Could you check a few things on this model? Use its own coordinates, in mm. Coordinates: 2 decimals unless noted, no trailing zeros. Loops run counter-clockwise (first coordinate to the right, second up) from the corner with the lowest first, then second, coordinate; pieces in that order, holes last. Notation, with made-up numbers: (6, 44) -> (26, 44) arc R24 cw to (26, 80) -> close; hole circle Ø10 at (40, -32). An arc over 180 degrees is marked (long way). One line per question, with ' | ' between items.
from build123d import *

# Parameters (mm, degrees)
BOSS_EXTRUDE1_DEPTH = 6
SKETCH2_R           = 3.25
CUT_EXTRUDE1_DEPTH  = 82.391031447
SKETCH3_R           = 5.5
CUT_EXTRUDE2_DEPTH  = 4.8


with BuildPart() as part:
    # Sketch1 → Boss-Extrude1 (new body)
    with BuildSketch(Plane(origin=(0, 0, 0), x_dir=(1, 0, 0), z_dir=(0, 1, 0))):
        with BuildLine():
            Line((-36.5, -72.5), (36.5, -72.5))
            Line((36.5, -72.5), (36.5, -24.5))
            Line((36.5, -24.5), (26.5, -24.5))
            ThreePointArc((26.5, -24.5), (22.964466094, -23.035533906), (21.5, -19.5))
            Line((21.5, -19.5), (21.5, 37.5))
            ThreePointArc((21.5, 37.5), (22.964466094, 41.035533906), (26.5, 42.5))
            Line((26.5, 42.5), (36.5, 42.5))
            Line((36.5, 42.5), (36.5, 72.5))
            Line((36.5, 72.5), (-36.5, 72.5))
            Line((-36.5, 72.5), (-36.5, 42.5))
            Line((-36.5, 42.5), (-26.5, 42.5))
            ThreePointArc((-26.5, 42.5), (-22.964466094, 41.035533906), (-21.5, 37.5))
            Line((-21.5, 37.5), (-21.5, -19.5))
            ThreePointArc((-21.5, -19.5), (-22.964466094, -23.035533906), (-26.5, -24.5))
            Line((-26.5, -24.5), (-36.5, -24.5))
            Line((-36.5, -24.5), (-36.5, -72.5))
        make_face()
    extrude(amount=BOSS_EXTRUDE1_DEPTH)

    # Sketch2 → Cut-Extrude1 (cut, through all)
    with BuildSketch(Plane(origin=(0, 6, 0), x_dir=(1, 0, 0), z_dir=(0, 1, 0))):
        with Locations(Location((-30, 66, 0), (0, 0, 270))):
            Circle(SKETCH2_R)
        with Locations(Location((-30, 50, 0), (0, 0, 270))):
            Circle(SKETCH2_R)
        with Locations(Location((30, 50, 0), (0, 0, 90))):
            Circle(SKETCH2_R)
        with Locations(Location((30, 66, 0), (0, 0, 90))):
            Circle(SKETCH2_R)
        with Locations(Location((30, -50, 0), (0, 0, 270))):
            Circle(SKETCH2_R)
        with Locations(Location((30, -66, 0), (0, 0, 270))):
            Circle(SKETCH2_R)
        with Locations(Location((-30, -50, 0), (0, 0, 90))):
            Circle(SKETCH2_R)
        with Locations(Location((-30, -66, 0), (0, 0, 90))):
            Circle(SKETCH2_R)
    extrude(amount=-CUT_EXTRUDE1_DEPTH, mode=Mode.SUBTRACT)

    # Sketch3 → Cut-Extrude2 (cut)
    with BuildSketch(Plane(origin=(0, 6, 0), x_dir=(1, 0, 0), z_dir=(0, 1, 0))):
        with Locations(Location((-30, 50, 0), (0, 0, 270))):
            Circle(SKETCH3_R)
        with Locations(Location((30, 50, 0), (0, 0, 90))):
            Circle(SKETCH3_R)
        with Locations(Location((30, -50, 0), (0, 0, 270))):
            Circle(SKETCH3_R)
        with Locations(Location((-30, -50, 0), (0, 0, 90))):
            Circle(SKETCH3_R)
    extrude(amount=-CUT_EXTRUDE2_DEPTH, mode=Mode.SUBTRACT)


solid = part.part
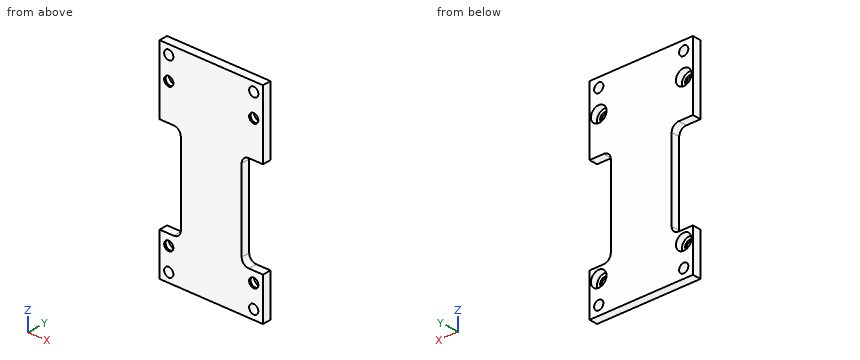
1) If we section it at D-D on z = 50: Please give me the cut outline in (x, y).
Data:
outline: (-36.5, 0) -> (-33.25, 0) -> (-33.25, 1.2) -> (-35.5, 1.2) -> (-35.5, 6) -> (-36.5, 6) -> close; (-26.75, 0) -> (26.75, 0) -> (26.75, 1.2) -> (24.5, 1.2) -> (24.5, 6) -> (-24.5, 6) -> (-24.5, 1.2) -> (-26.75, 1.2) -> close; (33.25, 0) -> (36.5, 0) -> (36.5, 6) -> (35.5, 6) -> (35.5, 1.2) -> (33.25, 1.2) -> close
2) If we section it at B-B on x = 30: Give the number of separate pieces and of enclosed holes in the cut face, and give its area (3 significant figures).
Data:
separate pieces: 6 | enclosed holes: 0 | area: 269 mm²
3) I need wall thicknesses on line 1 along X through (y, z) = (0.4, -50); line 2 along X through (y, z) = (3.6, 50); line 3 along Z through (x, y) = (25.5, 3.4). Which ranges of each line are inside material? Lowest first, please. Write a range as from..to.
Data:
line 1: -36.5..-33.25, -26.75..26.75, 33.25..36.5 | line 2: -36.5..-35.5, -24.5..24.5, 35.5..36.5 | line 3: -72.5..-53.16, -46.84..-42.4, 24.4..46.84, 53.16..72.5
4) If we section it at A-A on z = -66: Please give me the cut outline in (x, y).
Data:
outline: (-36.5, 0) -> (-33.25, 0) -> (-33.25, 6) -> (-36.5, 6) -> close; (-26.75, 0) -> (26.75, 0) -> (26.75, 6) -> (-26.75, 6) -> close; (33.25, 0) -> (36.5, 0) -> (36.5, 6) -> (33.25, 6) -> close
5) I'm going to push flat-ended pins straight in: pin 1 Ø5 at (x, z) = (30, 66) entering from -Y; pin 2 Ø1 at (y, z) = (5, -24) entering from +X; pin 3 Ø5.5 at (x, z) = (27.5, -50.5) entering from +Y. Where does each tip first touch, or does it pass through?
Data:
pin 1: through | pin 2: x = 21.5 | pin 3: y = 1.2
